from build123d import *

# Parameters (mm, degrees)
F0_W     = 132.08
F0_H     = 101.6
F1_DEPTH = 17.272
F3_DEPTH = 101.6
F6_DEPTH = 3.81


with BuildPart() as f1:
    # F0 (on Top) → F1 (new body)
    with BuildSketch(Plane.XY):
        with Locations((22.4865525961, 18.1711361257)):
            Rectangle(F0_W, F0_H)
    extrude(amount=F1_DEPTH)

    # F2 (on face) → F3 (join, through all)
    with BuildSketch(Plane.XZ.offset(32.6288638743)):
        with BuildLine():
            Line((-6.7586990196, 29.591), (-13.8706990196, 29.591))
            ThreePointArc((-13.8706990196, 29.591), (-17.4788505821, 20.8801515626), (-26.1896990196, 17.272))
            Line((-26.1896990196, 17.272), (5.560301017, 17.272))
            ThreePointArc((5.560301017, 17.272), (-3.1505474441, 20.8801515496), (-6.7586990196, 29.591))
        make_face()
        with BuildLine():
            ThreePointArc((-26.1896990196, 17.272), (-34.900547457, 20.8801515626), (-38.5086990196, 29.591))
            Line((-38.5086990196, 29.591), (-43.5534474039, 29.591))
            Line((-43.5534474039, 29.591), (-43.5534474039, 17.272))
            Line((-43.5534474039, 17.272), (-26.1896990196, 17.272))
        make_face()
        with BuildLine():
            ThreePointArc((17.8793009804, 29.591), (14.2711494308, 20.8801515755), (5.560301017, 17.272))
            Line((5.560301017, 17.272), (39.4128042118, 17.272))
            ThreePointArc((39.4128042118, 17.272), (30.7019557743, 20.8801515626), (27.0938042118, 29.591))
            Line((27.0938042118, 29.591), (17.8793009804, 29.591))
        make_face()
        with BuildLine():
            ThreePointArc((51.7318042118, 29.591), (48.1236526492, 20.8801515626), (39.4128042118, 17.272))
            Line((39.4128042118, 17.272), (71.1628042118, 17.272))
            ThreePointArc((71.1628042118, 17.272), (62.4519557743, 20.8801515626), (58.8438042118, 29.591))
            Line((58.8438042118, 29.591), (51.7318042118, 29.591))
        make_face()
        with BuildLine():
            ThreePointArc((83.4818042118, 29.591), (79.8736526492, 20.8801515626), (71.1628042118, 17.272))
            Line((71.1628042118, 17.272), (88.5265525961, 17.272))
            Line((88.5265525961, 17.272), (88.5265525961, 29.591))
            Line((88.5265525961, 29.591), (83.4818042118, 29.591))
        make_face()
    extrude(amount=-F3_DEPTH)

    # F5 (on face) → F6 (join)
    with BuildSketch(Plane.XZ.offset(32.6288638743)):
        with BuildLine():
            Line((-43.5534474039, 0), (88.5265525961, 0))
            Line((88.5265525961, 0), (88.5265525961, 29.591))
            Line((88.5265525961, 29.591), (83.4818042118, 29.591))
            ThreePointArc((83.4818042118, 29.591), (71.1628042118, 17.272), (58.8438042118, 29.591))
            Line((58.8438042118, 29.591), (51.7318042118, 29.591))
            ThreePointArc((51.7318042118, 29.591), (39.4128042118, 17.272), (27.0938042118, 29.591))
            Line((27.0938042118, 29.591), (17.8793009804, 29.591))
            ThreePointArc((17.8793009804, 29.591), (5.5603009804, 17.272), (-6.7586990196, 29.591))
            Line((-6.7586990196, 29.591), (-13.8706990196, 29.591))
            ThreePointArc((-13.8706990196, 29.591), (-26.1896990196, 17.272), (-38.5086990196, 29.591))
            Line((-38.5086990196, 29.591), (-43.5534474039, 29.591))
            Line((-43.5534474039, 29.591), (-43.5534474039, 0))
        make_face()
        with BuildLine():
            ThreePointArc((58.8438042118, 29.591), (71.1628042118, 17.272), (83.4818042118, 29.591))
            Line((83.4818042118, 29.591), (58.8438042118, 29.591))
        make_face()
        with BuildLine():
            Line((-13.8706990196, 29.591), (-38.5086990196, 29.591))
            ThreePointArc((-38.5086990196, 29.591), (-26.1896990196, 17.272), (-13.8706990196, 29.591))
        make_face()
        with BuildLine():
            ThreePointArc((27.0938042118, 29.591), (39.4128042118, 17.272), (51.7318042118, 29.591))
            Line((51.7318042118, 29.591), (27.0938042118, 29.591))
        make_face()
        with BuildLine():
            Line((17.8793009804, 29.591), (-6.7586990196, 29.591))
            ThreePointArc((-6.7586990196, 29.591), (5.5603009804, 17.272), (17.8793009804, 29.591))
        make_face()
    extrude(amount=F6_DEPTH)

    # F7: F1 across plane


with BuildPart() as f1_1:
    add(f1.part)
    add(f1.part.mirror(Plane(origin=(22.4865525961, 18.1711361257, 11.7082126405), x_dir=(1, 0, 0), z_dir=(0, -1, 0))))


solid = f1_1.part
Input: part model. Units: mm. Frame: model coordinates. A direction names the side the tool comes from. Give positions to 0.01 mm unless a question says otherwise; leave off trailing zeros. Order: outer loops, then holes, each group sorted by start corner. A loop starts at its lowest first (then second) coordinate and runs counter-clockwise, first axis right, second up. Notation, with made-up numbers: (52, 41.25) - (66, 41.25) arc R14 cw to (66, 51.25) - close; hole circle Ø4 at (50, 18.25). An arc over 180 degrees is marked (long way). Answer as a JSON object with one key per item and string values. Group by question number.
Q1. Cut plane C-C, the plane x = 34. Output: boundary loops of the cut face in (y, z), then the cut area to 3 significant figures.
Q2. Line query: probe 1 along Y at (x, z) = (-16.5, 26.75); probe 2 along X at (y, z) = (-5, 25); probe 3 along X at (y, z) = (-2, 21.5). Output: solid intervals per line, ascending.
Q3. Mould query, pull axis Y, two halves, no side actions, for faces 3 (the face through (22, 17, 0)), 4 (the face through (22, 72.781, 15)), 5 (the face through (39, -32.629, 25)). Classes: pulls with the +Y half, pulls with the -Y half, needs draft (parallel to the pull), parting line crosses it, or undercut.
Q4. Cut plane B-B, the plane z = 25. Output: boundary loops of the cut face in (x, y), then the cut area to 3 significant figures.
Q5. Cut plane A-A, the plane y = 13.5. Output: boundary loops of the cut face in (x, z), then the cut area to 3 significant figures.
Q6. Set-up query: faces 1 (the face through (5, -32.629, 25)), 2 (the face through (22, -36.439, 15)). Return all of +Z, -Z, +X, -X, +Y, -Y with unobstructed straight access to the full face (end or side cutting, diameter ignored); none if empty.
Q7. Cut plane D-D, the plane z = 18.75. Output: boundary loops of the cut face in (x, y).
Results:
{
 "1": {"outline": "(-36.44, 0) - (72.78, 0) - (72.78, 29.59) - (68.97, 29.59) - (68.97, 18.52) - (-32.63, 18.52) - (-32.63, 29.59) - (-36.44, 29.59) - close", "area": "2,110 mm^2"},
 "2": {"probe 1": "-36.44 to -32.63, 68.97 to 72.78", "probe 2": "-43.55 to -37.62, -14.76 to -5.87, 16.99 to 27.98, 50.84 to 59.73, 82.59 to 88.53", "probe 3": "-43.55 to -35.48, -16.9 to -3.73, 14.85 to 30.12, 48.7 to 61.87, 80.45 to 88.53"},
 "3": {"face 3": "needs draft", "face 4": "pulls with the +Y half", "face 5": "undercut"},
 "4": {"outline": "(-43.55, -36.44) - (88.53, -36.44) - (88.53, 72.78) - (-43.55, 72.78) - close; hole (-37.62, -32.63) - (-14.76, -32.63) - (-14.76, 68.97) - (-37.62, 68.97) - close; hole (-5.87, -32.63) - (16.99, -32.63) - (16.99, 68.97) - (-5.87, 68.97) - close; hole (27.98, -32.63) - (50.84, -32.63) - (50.84, 68.97) - (27.98, 68.97) - close; hole (59.73, -32.63) - (82.59, -32.63) - (82.59, 68.97) - (59.73, 68.97) - close", "area": "5,130 mm^2"},
 "5": {"outline": "(-43.55, 0) - (88.53, 0) - (88.53, 29.59) - (83.48, 29.59) arc R12.32 cw to (58.84, 29.59) - (51.73, 29.59) arc R12.32 cw to (27.09, 29.59) - (17.88, 29.59) arc R12.32 cw to (-6.76, 29.59) - (-13.87, 29.59) arc R12.32 cw to (-38.51, 29.59) - (-43.55, 29.59) - close", "area": "2,950 mm^2"},
 "6": {"face 1": "+Z", "face 2": "+Z, -Z, +X, -X, -Y"},
 "7": {"outline": "(-43.55, -36.44) - (88.53, -36.44) - (88.53, 72.78) - (-43.55, 72.78) - close; hole (-32.04, -32.63) - (-20.34, -32.63) - (-20.34, 68.97) - (-32.04, 68.97) - close; hole (-0.29, -32.63) - (11.41, -32.63) - (11.41, 68.97) - (-0.29, 68.97) - close; hole (33.56, -32.63) - (45.26, -32.63) - (45.26, 68.97) - (33.56, 68.97) - close; hole (65.31, -32.63) - (77.01, -32.63) - (77.01, 68.97) - (65.31, 68.97) - close"}
}
